Part model, mm, in its own coordinate system. Face numbers are marked on the shaded views. Round coordinates to 2 decimals unless told otherwise and drop trailing zeros. Loops run counter-clockwise (first coordinate to the right, second up) from the corner with the lowest first, then second, coordinate; pieces in that order, holes last. Notation, with made-up numbers: (60.5, 38.5) -> (80.5, 38.5) arc R13 ccw to (80.5, 60.5) -> close; hole circle Ø10 at (-2.5, 6). An arc over 180 degrees is marked (long way). Answer as CSV lines item,"result".
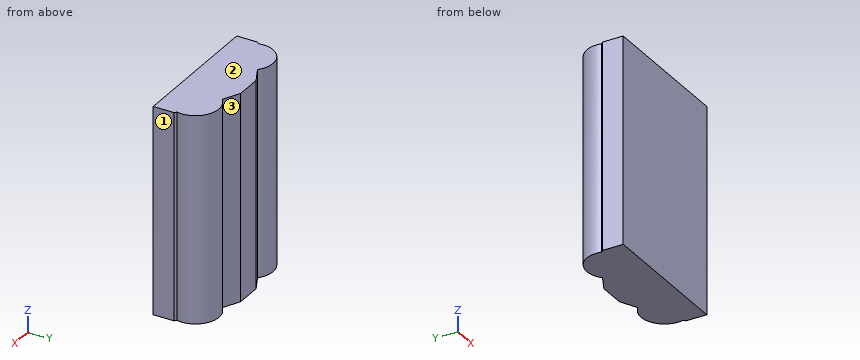
from build123d import *

# Parameters (mm, degrees)
SKETCH1_W           = 190
SKETCH1_H           = 278
BOSS_EXTRUDE1_DEPTH = 105
SKETCH3_OUTSIDE_W   = 262.544
SKETCH3_OUTSIDE_H   = 177.544
CUT_EXTRUDE1_DEPTH  = 353.71660012


with BuildPart() as part:
    # Sketch1 → Boss-Extrude1 (new body)
    with BuildSketch(Plane(origin=(0, 0, 0), x_dir=(1, 0, 0), z_dir=(0, 1, 0))):
        with Locations((95, 139)):
            Rectangle(SKETCH1_W, SKETCH1_H)
    extrude(amount=BOSS_EXTRUDE1_DEPTH)

    # Sketch3 outside → Cut-Extrude1 (cut, through all)
    with BuildSketch(Plane.XY):
        with Locations((95, 52.5)):
            Rectangle(SKETCH3_OUTSIDE_W, SKETCH3_OUTSIDE_H)
        with BuildLine():
            Line((54.836273007, 60.288293162), (77.499520746, 71.724132439))
            Line((77.499520746, 71.724132439), (112.500479254, 71.724132439))
            Line((112.500479254, 71.724132439), (135.163726993, 60.288293162))
            ThreePointArc((135.163726993, 60.288293162), (172.119968318, 64.39962656), (187.325162615, 30.466325783))
            Line((187.325162615, 30.466325783), (190, 27.791488398))
            Line((190, 27.791488398), (190, 0))
            Line((190, 0), (0, 0))
            Line((0, 0), (0, 27.791488398))
            Line((0, 27.791488398), (2.674837385, 30.466325783))
            ThreePointArc((2.674837385, 30.466325783), (17.880031682, 64.39962656), (54.836273007, 60.288293162))
        make_face(mode=Mode.SUBTRACT)
    extrude(amount=-CUT_EXTRUDE1_DEPTH, mode=Mode.SUBTRACT)


solid = part.part
Q1. Saw through at B-B, the plane y = 64.5. Write the cut outline in (x, z), then the cut area to 3 significant figures.
Geometry results:
outline,"(18.06, -278) -> (49.02, -278) -> (49.02, 0) -> (18.06, 0) -> close; (63.18, -278) -> (126.82, -278) -> (126.82, 0) -> (63.18, 0) -> close; (140.98, -278) -> (171.94, -278) -> (171.94, 0) -> (140.98, 0) -> close"
area,"34,900 mm2"
Q2. Saw through at D-D, the plane y = 43. Write the cut outline in (x, z), then the cut area to 3 significant figures.
Geometry results:
outline,"(2.56, -278) -> (187.44, -278) -> (187.44, 0) -> (2.56, 0) -> close"
area,"51,400 mm2"
Q3. Drill centre lines: line 1 along X through (y, z) = (64, -219.5); line 2 along X through (y, z) = (36.5, -92); line 3 along X through (y, z) = (30.5, -62.5). Where is each one in solid material? Low to high.
Geometry results:
line 1,"17.2 to 49.88, 62.19 to 127.81, 140.12 to 172.8"
line 2,"1.99 to 188.01"
line 3,"2.67 to 187.33"
Q4. Two-plate mould, pull along X, no slides. Class the marked faces 1, 2 and 3: pulls with the +X half, pulls with the -X half, needs draft (parallel to the pull), parting line crosses it, or undercut.
Geometry results:
face 1,"pulls with the +X half"
face 2,"needs draft"
face 3,"undercut"
Q5. Saw through at A-A, the plane z = -143.5. Write the cut outline in (x, y), then the cut area to 3 significant figures.
Geometry results:
outline,"(0, 0) -> (190, 0) -> (190, 27.79) -> (187.33, 30.47) arc R31.55 ccw to (135.16, 60.29) -> (112.5, 71.72) -> (77.5, 71.72) -> (54.84, 60.29) arc R31.55 ccw to (2.67, 30.47) -> (0, 27.79) -> close"
area,"12,300 mm2"
Q6. Saw through at C-C, the plane x = 70.5. Write the cut outline in (y, z), then the cut area to 3 significant figures.
Geometry results:
outline,"(0, -278) -> (68.19, -278) -> (68.19, 0) -> (0, 0) -> close"
area,"19,000 mm2"
Q7. Drop flat-ended pins along their axis: P1, Ø8, axis at y = 63, z = -116.5, coming from the +X side; P2, Ø3, axis at y = 36, z = -28.5, coming from the +X side; P3, Ø1.5, axis at x = 128.5, z = -85, coming from the +Y side. Give the stop position or say it passes through.
Geometry results:
P1,"x = 179.08"
P2,"x = 188.01"
P3,"y = 64.03"
